Input: part model. Units: mm. Frame: model coordinates. A direction names the side the tool comes from. Round coordinates to 2 decimals unless told otherwise and drop trailing zeros. Order: outer loops, then holes, each group sorted by start corner. A loop starts at its lowest first (then second) coordinate and runs counter-clockwise, first axis right, second up. Notation, with made-up numbers: M 37,56 L 63,56 A22 ccw 63,89 Z; hole C 19.5,68 d6. An arc over 180 degrees is marked long. One line per question, with ' | ' between items.
```python
from build123d import *

# Parameters (mm, degrees)
CYLINDER021_R          = 1.65
CYLINDER021_DEPTH      = 10
CYLINDER022_R          = 1.65
CYLINDER022_DEPTH      = 10
CYLINDER023_R          = 1.65
CYLINDER023_DEPTH      = 10
CYLINDER024_R          = 1.65
CYLINDER024_DEPTH      = 10
CYLINDER020_R          = 8.1
CYLINDER020_DEPTH      = 20
CYLINDER019_R          = 8.1
CYLINDER019_DEPTH      = 20
CYLINDER008_R          = 2.5
CYLINDER008_DEPTH      = 20
CYLINDER007_R          = 2.5
CYLINDER007_DEPTH      = 20
CYLINDER006_R          = 142
CYLINDER006_DEPTH      = 180
CYLINDER005_R          = 151
CYLINDER005_DEPTH      = 0.5
CYLINDER004_R          = 155
CYLINDER004_DEPTH      = 0.5
CUT002_PLACEMENT_ANGLE = 90
CYLINDER003_R          = 25
CYLINDER003_DEPTH      = 15
CYLINDER001_R          = 5
CYLINDER001_DEPTH      = 40
CYLINDER_R             = 4.2
CYLINDER_DEPTH         = 40
CYLINDER002_R          = 10
CYLINDER002_DEPTH      = 15
BOX001_W               = 70
BOX001_H               = 35
BOX001_DEPTH           = 50
BOX001_PLACEMENT_ANGLE = 69
BOX_W                  = 330
BOX_H                  = 35
BOX_DEPTH              = 330


with BuildPart() as zylinder021:
    # Cylinder021 → Cylinder021 (new body)
    with BuildSketch(Plane(origin=(25, 35, 25), x_dir=(1, 0, 0), z_dir=(0, -1, 0))):
        Circle(CYLINDER021_R)
    extrude(amount=CYLINDER021_DEPTH)


with BuildPart() as zylinder022:
    # Cylinder022 → Cylinder022 (new body)
    with BuildSketch(Plane(origin=(305, 35, 25), x_dir=(1, 0, 0), z_dir=(0, -1, 0))):
        Circle(CYLINDER022_R)
    extrude(amount=CYLINDER022_DEPTH)


with BuildPart() as zylinder023:
    # Cylinder023 → Cylinder023 (new body)
    with BuildSketch(Plane(origin=(25, 35, 305), x_dir=(1, 0, 0), z_dir=(0, -1, 0))):
        Circle(CYLINDER023_R)
    extrude(amount=CYLINDER023_DEPTH)


with BuildPart() as obj1:
    # Cylinder024 → Cylinder024 (new body)
    with BuildSketch(Plane(origin=(305, 35, 305), x_dir=(1, 0, 0), z_dir=(0, -1, 0))):
        Circle(CYLINDER024_R)
    extrude(amount=CYLINDER024_DEPTH)

    # Fusion006: union Zylinder021, Zylinder022, Zylinder023
    add(zylinder021.part)
    add(zylinder022.part)
    add(zylinder023.part)


with BuildPart() as zylinder020:
    # Cylinder020 → Cylinder020 (new body)
    with BuildSketch(Plane(origin=(80, 1, 40), x_dir=(1, 0, 0), z_dir=(0, -1, 0))):
        Circle(CYLINDER020_R)
    extrude(amount=CYLINDER020_DEPTH)


with BuildPart() as fusion005:
    # Cylinder019 → Cylinder019 (new body)
    with BuildSketch(Plane(origin=(250, 1, 40), x_dir=(1, 0, 0), z_dir=(0, -1, 0))):
        Circle(CYLINDER019_R)
    extrude(amount=CYLINDER019_DEPTH)

    # Fusion005: union Zylinder020
    add(zylinder020.part)


with BuildPart() as zylinder008:
    # Cylinder008 → Cylinder008 (new body)
    with BuildSketch(Plane(origin=(250, 20, 40), x_dir=(1, 0, 0), z_dir=(0, -1, 0))):
        Circle(CYLINDER008_R)
    extrude(amount=CYLINDER008_DEPTH)


with BuildPart() as fusion003:
    # Cylinder007 → Cylinder007 (new body)
    with BuildSketch(Plane(origin=(80, 20, 40), x_dir=(1, 0, 0), z_dir=(0, -1, 0))):
        Circle(CYLINDER007_R)
    extrude(amount=CYLINDER007_DEPTH)

    # Fusion003: union Zylinder008
    add(zylinder008.part)


with BuildPart() as zylinder006:
    # Cylinder006 → Cylinder006 (new body)
    with BuildSketch(Plane(origin=(165, 200, 165), x_dir=(1, 0, 0), z_dir=(0, -1, 0))):
        Circle(CYLINDER006_R)
    extrude(amount=CYLINDER006_DEPTH)


with BuildPart() as zylinder005:
    # Cylinder005 → Cylinder005 (new body)
    with BuildSketch(Plane.XY):
        Circle(CYLINDER005_R)
    extrude(amount=CYLINDER005_DEPTH)


with BuildPart() as cut002:
    # Cylinder004 → Cylinder004 (new body)
    with BuildSketch(Plane.XY):
        Circle(CYLINDER004_R)
    extrude(amount=CYLINDER004_DEPTH)

    # Cut002: cut Zylinder005
    add(zylinder005.part, mode=Mode.SUBTRACT)


with BuildPart() as cut002_1:
    # Cut002 placement: moved
    add(cut002.part.moved(Location((165, 35, 165))).rotate(Axis((165, 35, 165), (1, 0, 0)), CUT002_PLACEMENT_ANGLE))


with BuildPart() as zylinder003:
    # Cylinder003 → Cylinder003 (new body)
    with BuildSketch(Plane(origin=(36, 0, 34), x_dir=(1, 0, 0), z_dir=(0, 1, 0))):
        Circle(CYLINDER003_R)
    extrude(amount=CYLINDER003_DEPTH)


with BuildPart() as fusion001:
    # Cylinder001 → Cylinder001 (new body)
    with BuildSketch(Plane(origin=(36, 0, 34), x_dir=(1, 0, 0), z_dir=(0, 1, 0))):
        Circle(CYLINDER001_R)
    extrude(amount=CYLINDER001_DEPTH)

    # Fusion001: union Zylinder003
    add(zylinder003.part)


with BuildPart() as zylinder:
    # Cylinder → Cylinder (new body)
    with BuildSketch(Plane(origin=(302, 0, 34), x_dir=(1, 0, 0), z_dir=(0, 1, 0))):
        Circle(CYLINDER_R)
    extrude(amount=CYLINDER_DEPTH)


with BuildPart() as fusion002:
    # Cylinder002 → Cylinder002 (new body)
    with BuildSketch(Plane(origin=(302, 0, 34), x_dir=(1, 0, 0), z_dir=(0, 1, 0))):
        Circle(CYLINDER002_R)
    extrude(amount=CYLINDER002_DEPTH)

    # Fusion: union Zylinder
    add(zylinder.part)

    # Fusion002: union Fusion001
    add(fusion001.part)


with BuildPart() as obj2:
    # Box001 → Box001 (new body)
    with BuildSketch(Plane.XY):
        with Locations((35, 17.5)):
            Rectangle(BOX001_W, BOX001_H)
    extrude(amount=BOX001_DEPTH)


with BuildPart() as obj2_1:
    # Box001 placement: moved
    add(obj2.part.moved(Location((0, 0, 265))).rotate(Axis((0, 0, 265), (0, -1, 0)), BOX001_PLACEMENT_ANGLE))


with BuildPart() as simplefrontdoor01:
    # Box → Box (new body)
    with BuildSketch(Plane.XY):
        with Locations((165, 17.5)):
            Rectangle(BOX_W, BOX_H)
    extrude(amount=BOX_DEPTH)

    # Cut: cut obj2
    add(obj2_1.part, mode=Mode.SUBTRACT)

    # Cut001: cut Fusion002
    add(fusion002.part, mode=Mode.SUBTRACT)

    # Cut003: cut Cut002
    add(cut002_1.part, mode=Mode.SUBTRACT)

    # Cut004: cut Zylinder006
    add(zylinder006.part, mode=Mode.SUBTRACT)

    # Cut005: cut Fusion003
    add(fusion003.part, mode=Mode.SUBTRACT)

    # Cut011: cut Fusion005
    add(fusion005.part, mode=Mode.SUBTRACT)

    # Cut012: cut obj1
    add(obj1.part, mode=Mode.SUBTRACT)


solid = simplefrontdoor01.part
```
Item 1: Line query: line 1 along X through (y, z) = (5.5, 34); line 2 along Z through (x, y) = (80, 5); line 3 along Z through (x, y) = (165, 25). Output: solid intervals per line, ascending. Write a range as from..to.
Report:
line 1: 0..11, 61..292, 312..330 | line 2: 0..37.5, 42.5..330 | line 3: 0..23, 307..330
Item 2: Section query B-B, the plane z = 165. Return loops of the section in (x, y).
Report:
outline: M 0,0 L 330,0 L 330,35 L 320,35 L 320,34.5 L 316,34.5 L 316,35 L 307,35 L 307,20 L 23,20 L 23,35 L 14,35 L 14,34.5 L 10,34.5 L 10,35 L 0,35 Z
Item 3: Mould query, pull axis X, two halves, no side actions, for faces 1 (the cylindrical face through (146.51, 27.6, 305.79)), 2 (the flat face through (12.3, 17.74, 297.04)), 3 (the flat face through (276, 35, 254)), 4 (the flat face through (330, 17, 163)). Classes: +X half, -X half, draft (parallel to the pull), parting line (faces both ways), or undercut.
Report:
face 1: undercut | face 2: -X half | face 3: draft | face 4: +X half
Item 4: First-contact query: pin 1 (4 mm diameter, centred on x = 86.5, z = 164, fed in from +Y); pin 2 (2 mm diameter, centred on x = 25, z = 25, fed in from +Y); pin 3 (6.5 mm diameter, centred on x = 250, z = 40, fed in from -Y). Flat tips, straight axial feed; report the tip coordinate or a pass-through.
Report:
pin 1: y = 20 | pin 2: y = 25 | pin 3: y = 1
Item 5: Access query for faces 5 (the cylindrical face through (10.15, 34.75, 171.82)), 6 (the cylindrical face through (257.482, 0.507, 36.898)), 7 (the cylindrical face through (306.006, 24.86, 32.738)). Directions: +Z, -Z, +X, -X, +Y, -Y. A direction counts if a zero-diameter tool reaches every point of the face in a straight line with its end or side. Return the directions, or none.
Report:
face 5: +Y | face 6: -Y | face 7: +Y, -Y
Item 6: Section query A-A, the plane x = 165. Return loops of the section in (y, z), plus the area to 3 significant figures.
Report:
outline: M 0,0 L 35,0 L 35,10 L 34.5,10 L 34.5,14 L 35,14 L 35,23 L 20,23 L 20,307 L 35,307 L 35,316 L 34.5,316 L 34.5,320 L 35,320 L 35,330 L 0,330 Z | area: 7,290 mm²
